Read the model definition and answer for the solid it produces. Units are mm, in the model's axes. A direction names the side the tool comes from. Round coordinates to 2 decimals unless told otherwise and drop trailing zeros. Write each loop counter-clockwise with the first axis right and the second up, starting at its lowest first coordinate (ties: lowest second). Pieces come first, ordered by that corner, then holes. Notation, with made-up numbers: (56.5, 29.5) -> (82.5, 29.5) arc R25 cw to (82.5, 45.5) -> close; hole circle Ø7 at (-28, 41). An arc over 180 degrees is marked (long way). Return JSON: item names as keys, results as strings.
from build123d import *

# Parameters (mm, degrees)
ESQUISSE1_R        = 10.7
BOSS_EXTRU_1_DEPTH = 61
ESQUISSE2_R        = 18.25
BOSS_EXTRU_2_DEPTH = 150
ESQUISSE3_R        = 1
BOSS_EXTRU_3_DEPTH = 10


with BuildPart() as part:
    # Esquisse1 → Boss.-Extru.1 (new body)
    with BuildSketch(Plane(origin=(0, 0, 0), x_dir=(1, 0, 0), z_dir=(0, 1, 0))):
        Circle(ESQUISSE1_R)
    extrude(amount=-BOSS_EXTRU_1_DEPTH)

    # Esquisse2 → Boss.-Extru.2 (add)
    with BuildSketch(Plane(origin=(0, 0, 0), x_dir=(1, 0, 0), z_dir=(0, 1, 0))):
        Circle(ESQUISSE2_R)
    extrude(amount=BOSS_EXTRU_2_DEPTH)

    # Esquisse3 → Boss.-Extru.3 (add)
    with BuildSketch(Plane.XZ.offset(61)):
        Circle(ESQUISSE3_R)
    extrude(amount=BOSS_EXTRU_3_DEPTH)

    # Esquisse4 → Enlèvement de matière-Révolution1 (revolve, cut)
    with BuildSketch(Plane.XY):
        with BuildLine():
            Line((18.25, 21.5), (18.25, 24.5))
            ThreePointArc((18.25, 24.5), (16.75, 23), (18.25, 21.5))
        make_face()
    revolve(axis=Axis((0, 150, 0), (0, -1, 0)), mode=Mode.SUBTRACT)


solid = part.part
Item 1: Straight lines are drawn through the part: L1, parallel to Y at x = 6, z = -17; L2, parallel to Y at x = 14, z = 4.5; L3, parallel to Z at x = 0, y = -11. For each, find the intervals that lie inside material, in ascending order. Write a range as [from, to].
Worked answers:
{"L1": "y = [0, 21.52], [24.48, 150]", "L2": "y = [0, 150]", "L3": "z = [-10.7, 10.7]"}
Item 2: Flat-ended cylindrical pins translate along their axes: pin 1 (8 mm diameter, centred on y = -46.5, z = 8.5, fed in from +X); pin 2 (2 mm diameter, centred on x = -9.5, z = 3.5, fed in from -Y); pin 3 (5 mm diameter, centred on x = 9, y = 12, fed in from -Z). Find the tip coordinate at first contact, or state that the pin passes through.
Worked answers:
{"pin 1": "stops at x = 9.71", "pin 2": "stops at y = -61", "pin 3": "stops at z = -17.05"}
Item 3: A tool of negligible diameter and unlimited length cuts with its end or side. For faces 1 (the flat face through (8, 0, 8)), 2 (the flat face through (0, 150, 0)), from which of +Z, -Z, +X, -X, +Y, -Y can it reach the whole face along a straight path? Write none if from no direction.
Worked answers:
{"face 1": "-Y", "face 2": "+Z, -Z, +X, -X, +Y"}
Item 4: Section A-A (y = 98) is taken. Give the vertices of the cut face in (x, z), then the cut area to 3 significant figures.
Worked answers:
{"outline": "circle Ø36.5 at (0, 0)", "area": "1,050 mm2"}
